Could you check a few things on this model? Use its own coordinates, in mm. A direction names the side the tool comes from. Round coordinates to 2 decimals unless told otherwise and drop trailing zeros. Write each loop counter-clockwise with the first axis right and the second up, starting at its lowest first coordinate (ties: lowest second). Pieces come first, ordered by that corner, then holes.
```python
from build123d import *

# Parameters (mm, degrees)
F0_R     = 4.75
F1_DEPTH = 20
F2_DEPTH = 10
F3_R     = 13
F4_DEPTH = 25


with BuildPart() as f1:
    # F0 (on Top) → F1 (new body)
    with BuildSketch(Plane.XY):
        with BuildLine():
            Line((-8.6448206271, 31.9791635871), (-8.6448206271, 41.9791635871))
            ThreePointArc((-8.6448206271, 41.9791635871), (-14.4995413925, 41.6352029455), (-20.2737104175, 40.6080533775))
            Line((-20.2737104175, 40.6080533775), (-13.6448206271, 33.9791635871))
            Line((-13.6448206271, 33.9791635871), (-23.6448206271, 33.9791635871))
            Line((-23.6448206271, 33.9791635871), (-23.6448206271, 39.6761236579))
            ThreePointArc((-23.6448206271, 39.6761236579), (-26.1698127892, 38.8073030944), (-28.6448206271, 37.8049205367))
            Line((-28.6448206271, 37.8049205367), (-28.6448206271, -28.0208364129))
            Line((-28.6448206271, -28.0208364129), (-8.6448206271, -28.0208364129))
            Line((-8.6448206271, -28.0208364129), (35.0765389229, -28.0208364129))
            Line((35.0765389229, -28.0208364129), (36.0765389229, -28.0208364129))
            Line((36.0765389229, -28.0208364129), (36.0765389229, -7.0208364129))
            ThreePointArc((36.0765389229, -7.0208364129), (35.783645704, -7.7279431941), (35.0765389229, -8.0208364129))
            Line((35.0765389229, -8.0208364129), (31.3551793729, -8.0208364129))
            ThreePointArc((31.3551793729, -8.0208364129), (3.0709081254, 3.6948923396), (-8.6448206271, 31.9791635871))
        make_face()
        with Locations((-18.6448206271, -18.0208364129)):
            Circle(F0_R, mode=Mode.SUBTRACT)
        Polygon((-0.6448206271, -13.0208364129), (9.3551793729, -13.0208364129), (-0.6448206271, -23.0208364129), align=None, mode=Mode.SUBTRACT)
        Polygon((26.3551793729, -23.0208364129), (16.3551793729, -23.0208364129), (26.3551793729, -13.0208364129), align=None, mode=Mode.SUBTRACT)
        Polygon((-23.6448206271, -0.0208364129), (-23.6448206271, 9.9791635871), (-13.6448206271, -0.0208364129), align=None, mode=Mode.SUBTRACT)
        Polygon((-13.6448206271, 26.9791635871), (-13.6448206271, 16.9791635871), (-23.6448206271, 26.9791635871), align=None, mode=Mode.SUBTRACT)
        with BuildLine():
            Line((-8.6448206271, 41.9791635871), (-8.6448206271, 51.9791635871))
            ThreePointArc((-8.6448206271, 51.9791635871), (-18.7909393507, 51.1150771663), (-28.6448206271, 48.547706082))
            Line((-28.6448206271, 48.547706082), (-28.6448206271, 37.8049205367))
            ThreePointArc((-28.6448206271, 37.8049205367), (-26.1698127892, 38.8073030944), (-23.6448206271, 39.6761236579))
            Line((-23.6448206271, 39.6761236579), (-23.6448206271, 43.9791635871))
            Line((-23.6448206271, 43.9791635871), (-20.2737104175, 40.6080533775))
            ThreePointArc((-20.2737104175, 40.6080533775), (-14.4995413925, 41.6352029455), (-8.6448206271, 41.9791635871))
        make_face()
        with BuildLine():
            Line((-8.6448206271, 51.9791635871), (-8.6448206271, 61.9791635871))
            ThreePointArc((-8.6448206271, 61.9791635871), (-12.0320760881, 61.8971619884), (-15.4113955387, 61.651349314))
            ThreePointArc((-15.4113955387, 61.651349314), (-18.1852012194, 58.7618277327), (-21.6571207156, 60.7591028602))
            ThreePointArc((-21.6571207156, 60.7591028602), (-25.1727879958, 59.9999419909), (-28.6448206271, 59.0612029121))
            Line((-28.6448206271, 59.0612029121), (-28.6448206271, 48.547706082))
            ThreePointArc((-28.6448206271, 48.547706082), (-18.7909393507, 51.1150771663), (-8.6448206271, 51.9791635871))
        make_face()
        with BuildLine():
            Line((-8.6448206271, 61.9791635871), (-8.6448206271, 71.9791635871))
            ThreePointArc((-8.6448206271, 71.9791635871), (-18.7251640258, 71.3415392885), (-28.6448206271, 69.4388305112))
            Line((-28.6448206271, 69.4388305112), (-28.6448206271, 59.0612029121))
            ThreePointArc((-28.6448206271, 59.0612029121), (-25.1727879958, 59.9999419909), (-21.6571207156, 60.7591028602))
            ThreePointArc((-21.6571207156, 60.7591028602), (-19.2663207127, 65.1691851613), (-15.3948206271, 61.9791635871))
            ThreePointArc((-15.3948206271, 61.9791635871), (-15.398967, 61.8150470695), (-15.4113955387, 61.651349314))
            ThreePointArc((-15.4113955387, 61.651349314), (-12.0320760881, 61.8971619884), (-8.6448206271, 61.9791635871))
        make_face()
        with BuildLine():
            ThreePointArc((-28.6448206271, 69.4388305112), (-18.7251640258, 71.3415392885), (-8.6448206271, 71.9791635871))
            Line((-8.6448206271, 71.9791635871), (-28.6448206271, 71.9791635871))
            Line((-28.6448206271, 71.9791635871), (-28.6448206271, 69.4388305112))
        make_face()
        with BuildLine():
            ThreePointArc((60.6372116756, 31.9791635871), (31.3551793729, 61.2611958898), (-8.6448206271, 71.9791635871))
            Line((-8.6448206271, 71.9791635871), (-8.6448206271, 61.9791635871))
            ThreePointArc((-8.6448206271, 61.9791635871), (23.7588828649, 54.027531817), (48.8008058382, 31.9791635871))
            Line((48.8008058382, 31.9791635871), (60.6372116756, 31.9791635871))
        make_face()
        with BuildLine():
            ThreePointArc((36.0765389229, 31.9791635871), (15.8500768007, 46.7514193376), (-8.6448206271, 51.9791635871))
            Line((-8.6448206271, 51.9791635871), (-8.6448206271, 41.9791635871))
            ThreePointArc((-8.6448206271, 41.9791635871), (17.6417349788, 34.5117040047), (36.0765389229, 14.3398433621))
            Line((36.0765389229, 14.3398433621), (36.0765389229, 31.9791635871))
        make_face()
        with BuildLine():
            ThreePointArc((51.3551793729, -8.0208364129), (47.4055209106, 13.3884889735), (36.0765389229, 31.9791635871))
            Line((36.0765389229, 31.9791635871), (36.0765389229, 14.3398433621))
            ThreePointArc((36.0765389229, 14.3398433621), (40.0176288462, 3.4668096145), (41.3551793729, -8.0208364129))
            ThreePointArc((41.3551793729, -8.0208364129), (40.0176288462, -19.5084824403), (36.0765389229, -30.3815161879))
            Line((36.0765389229, -30.3815161879), (36.0765389229, -48.0208364129))
            ThreePointArc((36.0765389229, -48.0208364129), (47.4055209106, -29.4301617993), (51.3551793729, -8.0208364129))
        make_face()
        with BuildLine():
            ThreePointArc((61.3367884406, -6.4163451244), (57.898239576, 13.70521106), (48.8008058382, 31.9791635871))
            Line((48.8008058382, 31.9791635871), (36.0765389229, 31.9791635871))
            ThreePointArc((36.0765389229, 31.9791635871), (47.4055209106, 13.3884889735), (51.3551793729, -8.0208364129))
            ThreePointArc((51.3551793729, -8.0208364129), (47.4055209106, -29.4301617993), (36.0765389229, -48.0208364129))
            Line((36.0765389229, -48.0208364129), (48.8008058382, -48.0208364129))
            ThreePointArc((48.8008058382, -48.0208364129), (57.898239576, -29.7468838858), (61.3367884406, -9.6253277014))
            ThreePointArc((61.3367884406, -9.6253277014), (60.9015389229, -8.0208364129), (61.3367884406, -6.4163451244))
        make_face()
        with BuildLine():
            ThreePointArc((71.0765389229, -1.3496422544), (67.697860886, 15.891398518), (60.6372116756, 31.9791635871))
            Line((60.6372116756, 31.9791635871), (48.8008058382, 31.9791635871))
            ThreePointArc((48.8008058382, 31.9791635871), (57.898239576, 13.70521106), (61.3367884406, -6.4163451244))
            ThreePointArc((61.3367884406, -6.4163451244), (64.9077781239, -4.9565801588), (67.2515389229, -8.0208364129))
            ThreePointArc((67.2515389229, -8.0208364129), (64.9077781239, -11.085092667), (61.3367884406, -9.6253277014))
            ThreePointArc((61.3367884406, -9.6253277014), (57.898239576, -29.7468838858), (48.8008058382, -48.0208364129))
            Line((48.8008058382, -48.0208364129), (60.6372116756, -48.0208364129))
            ThreePointArc((60.6372116756, -48.0208364129), (67.697860886, -31.9330713438), (71.0765389229, -14.6920305714))
            Line((71.0765389229, -14.6920305714), (71.0765389229, -1.3496422544))
        make_face()
        with BuildLine():
            Line((71.0765389229, 31.9791635871), (60.6372116756, 31.9791635871))
            ThreePointArc((60.6372116756, 31.9791635871), (67.697860886, 15.891398518), (71.0765389229, -1.3496422544))
            Line((71.0765389229, -1.3496422544), (71.0765389229, 31.9791635871))
        make_face()
        with BuildLine():
            ThreePointArc((41.3551793729, -8.0208364129), (40.0176288462, 3.4668096145), (36.0765389229, 14.3398433621))
            Line((36.0765389229, 14.3398433621), (36.0765389229, -7.0208364129))
            Line((36.0765389229, -7.0208364129), (36.0765389229, -28.0208364129))
            Line((36.0765389229, -28.0208364129), (36.0765389229, -29.0208364129))
            Line((36.0765389229, -29.0208364129), (36.0765389229, -30.3815161879))
            ThreePointArc((36.0765389229, -30.3815161879), (40.0176288462, -19.5084824403), (41.3551793729, -8.0208364129))
        make_face()
        with BuildLine():
            ThreePointArc((71.0765389229, -14.6920305714), (67.697860886, -31.9330713438), (60.6372116756, -48.0208364129))
            Line((60.6372116756, -48.0208364129), (71.0765389229, -48.0208364129))
            Line((71.0765389229, -48.0208364129), (71.0765389229, -14.6920305714))
        make_face()
    extrude(amount=F1_DEPTH)

    # F0 (on Top) → F2 (join)
    with BuildSketch(Plane.XY):
        with BuildLine():
            ThreePointArc((41.3551793729, -8.0208364129), (40.0176288462, 3.4668096145), (36.0765389229, 14.3398433621))
            Line((36.0765389229, 14.3398433621), (36.0765389229, -7.0208364129))
            Line((36.0765389229, -7.0208364129), (36.0765389229, -28.0208364129))
            Line((36.0765389229, -28.0208364129), (36.0765389229, -29.0208364129))
            Line((36.0765389229, -29.0208364129), (36.0765389229, -30.3815161879))
            ThreePointArc((36.0765389229, -30.3815161879), (40.0176288462, -19.5084824403), (41.3551793729, -8.0208364129))
        make_face()
        with BuildLine():
            ThreePointArc((51.3551793729, -8.0208364129), (47.4055209106, 13.3884889735), (36.0765389229, 31.9791635871))
            Line((36.0765389229, 31.9791635871), (36.0765389229, 14.3398433621))
            ThreePointArc((36.0765389229, 14.3398433621), (40.0176288462, 3.4668096145), (41.3551793729, -8.0208364129))
            ThreePointArc((41.3551793729, -8.0208364129), (40.0176288462, -19.5084824403), (36.0765389229, -30.3815161879))
            Line((36.0765389229, -30.3815161879), (36.0765389229, -48.0208364129))
            ThreePointArc((36.0765389229, -48.0208364129), (47.4055209106, -29.4301617993), (51.3551793729, -8.0208364129))
        make_face()
        with BuildLine():
            ThreePointArc((61.3367884406, -6.4163451244), (57.898239576, 13.70521106), (48.8008058382, 31.9791635871))
            Line((48.8008058382, 31.9791635871), (36.0765389229, 31.9791635871))
            ThreePointArc((36.0765389229, 31.9791635871), (47.4055209106, 13.3884889735), (51.3551793729, -8.0208364129))
            ThreePointArc((51.3551793729, -8.0208364129), (47.4055209106, -29.4301617993), (36.0765389229, -48.0208364129))
            Line((36.0765389229, -48.0208364129), (48.8008058382, -48.0208364129))
            ThreePointArc((48.8008058382, -48.0208364129), (57.898239576, -29.7468838858), (61.3367884406, -9.6253277014))
            ThreePointArc((61.3367884406, -9.6253277014), (60.9015389229, -8.0208364129), (61.3367884406, -6.4163451244))
        make_face()
        with BuildLine():
            ThreePointArc((71.0765389229, -1.3496422544), (67.697860886, 15.891398518), (60.6372116756, 31.9791635871))
            Line((60.6372116756, 31.9791635871), (48.8008058382, 31.9791635871))
            ThreePointArc((48.8008058382, 31.9791635871), (57.898239576, 13.70521106), (61.3367884406, -6.4163451244))
            ThreePointArc((61.3367884406, -6.4163451244), (64.9077781239, -4.9565801588), (67.2515389229, -8.0208364129))
            ThreePointArc((67.2515389229, -8.0208364129), (64.9077781239, -11.085092667), (61.3367884406, -9.6253277014))
            ThreePointArc((61.3367884406, -9.6253277014), (57.898239576, -29.7468838858), (48.8008058382, -48.0208364129))
            Line((48.8008058382, -48.0208364129), (60.6372116756, -48.0208364129))
            ThreePointArc((60.6372116756, -48.0208364129), (67.697860886, -31.9330713438), (71.0765389229, -14.6920305714))
            Line((71.0765389229, -14.6920305714), (71.0765389229, -1.3496422544))
        make_face()
        with BuildLine():
            Line((71.0765389229, 31.9791635871), (60.6372116756, 31.9791635871))
            ThreePointArc((60.6372116756, 31.9791635871), (67.697860886, 15.891398518), (71.0765389229, -1.3496422544))
            Line((71.0765389229, -1.3496422544), (71.0765389229, 31.9791635871))
        make_face()
        with BuildLine():
            ThreePointArc((71.0765389229, -14.6920305714), (67.697860886, -31.9330713438), (60.6372116756, -48.0208364129))
            Line((60.6372116756, -48.0208364129), (71.0765389229, -48.0208364129))
            Line((71.0765389229, -48.0208364129), (71.0765389229, -14.6920305714))
        make_face()
    extrude(amount=-F2_DEPTH)

    # F3 (on face) → F4 (cut)
    with BuildSketch(Plane.YZ.offset(71.0765389229)):
        with Locations((-8.0208364129, 5)):
            Circle(F3_R)
    extrude(amount=-F4_DEPTH, mode=Mode.SUBTRACT)


solid = f1.part
```
Q1. Imagine slicing it at D-D, the plane x = 58.5. Write out the boundary of the cut face in (y, z).
Q2. I'm going to push flat-ended pins straight in: pin 1 Ø3 at (y, z) = (56.5, 10.5) entering from +X; pin 2 Ø4 at (y, z) = (-30.5, -5) entering from -X; pin 3 Ø8 at (x, z) = (60, -0.5) entering from +Y. Where does each tip first touch, or does it pass through?
Q3. Imagine slicing it at C-C, the plane y = 19.5. Write out the boundary of the cut face in (x, z).
Q4. If I drill on L1, parallel to X at y = -17.5, z = 0.5; L2, parallel to Y at x = 18.5, z = 19.5; L3, parallel to Y at x = 19.5, z = 2, over which ranges is the centre line in solid material (lowest first)?
Q5. Imagine slicing it at B-B, the plane x = 28.5. Write out the boundary of the cut face in (y, z), then the cut area to 3 significant figures.
Q6. We'd pull the mould along Y, two halves only. Please class faces 4 (the flat face through (-19, 26.979, 10)), 5 (the flat face through (32, 26, 20)), 6 (the flat face through (53, -48.021, 5)), 7 (the cylindrical face through (16.172, 46.606, 9.86)): pulls with the +Y half, pulls with the -Y half, needs draft (parallel to the pull), parting line crosses it, or undercut.
Q7. On a 3-axis mill with a long thin cutter (end or side, diameter ignored), from which of +Z, -Z, +X, -X, +Y, -Y can I reach the whole of each face in a straight line? I mean faces 1 (the flat face through (54, 31.979, -1)), 2 (the flat face through (-8.645, 37, 10)), 3 (the flat face through (3, -28.021, 10)). Say none if no direction works.
Q8. Imagine slicing it at A-A, the plane y = 40. Write out the boundary of the cut face in (x, z), then the cut area to 3 significant figures.
Results found:
1. outline: (-48.02, -10) - (31.98, -10) - (31.98, 0) - (35.47, 0) - (35.47, 20) - (-48.02, 20) - close; hole circle Ø26 at (-8.02, 5)
2. pin 1: stops at x = 40.63
2. pin 2: stops at x = 36.08
2. pin 3: stops at y = 39.06
3. outline: (-28.64, 0) - (-16.17, 0) - (-16.17, 20) - (-28.64, 20) - close; (-13.64, 0) - (-6.65, 0) - (-6.65, 20) - (-13.64, 20) - close; (33.1, 0) - (36.08, 0) - (36.08, -10) - (71.08, -10) - (71.08, 20) - (33.1, 20) - close
4. L1: x = -28.64 to -23.37, -13.92 to -0.64, 4.88 to 21.88, 26.36 to 46.08
4. L2: y = -28.02 to -23.02, -20.88 to -5.9, 33.97 to 45.49, 56.5 to 67.23
4. L3: y = -28.02 to -23.02, -19.88 to -6.22, 33.31 to 44.97, 56.07 to 66.86
5. outline: (-28.02, 0) - (-7.92, 0) - (-7.92, 20) - (-28.02, 20) - close; (25.45, 0) - (39.1, 0) - (39.1, 20) - (25.45, 20) - close; (51.31, 0) - (62.83, 0) - (62.83, 20) - (51.31, 20) - close
5. area: 905 mm2
6. face 4: undercut
6. face 5: needs draft
6. face 6: pulls with the -Y half
6. face 7: undercut
7. face 1: -Z
7. face 2: +Z, -Z
7. face 3: +Z, -Z, -X, -Y
8. outline: (-28.64, 0) - (-23.64, 0) - (-23.64, 20) - (-28.64, 20) - close; (-19.67, 0) - (-8.64, 0) - (-8.64, 20) - (-19.67, 20) - close; (5.28, 0) - (27.33, 0) - (27.33, 20) - (5.28, 20) - close; (42.29, 0) - (55.34, 0) - (55.34, 20) - (42.29, 20) - close
8. area: 1,020 mm2
